Geometry: final body of the model. Coordinates: model frame, mm. Face numbers are marked on the shaded views. A direction names the side the tool comes from. Round coordinates to 2 decimals unless told otherwise and drop trailing zeros. Order: outer loops, then holes, each group sorted by start corner. A loop starts at its lowest first (then second) coordinate and runs counter-clockwise, first axis right, second up. Notation, with made-up numbers: (40, -17.75) - (81, -17.75) arc R9 ccw to (81, -3.75) - close; hole circle Ø5 at (0, 8.25). An arc over 180 degrees is marked (long way). Put each result on its own line as item: value. Start each with the question number.
(1) Section B-B (x = 10). Output: boundary loops of the cut face in (y, z), and give its area (3 significant figures).
(2) Access query for the marked faces 1, 2 and 3. Directions: +Z, -Z, +X, -X, +Y, -Y. A direction counts if a zero-diameter tool reaches every point of the face in a straight line with its end or side. Return the directions, or none.
(3) Section C-C (y = 4.75). Output: boundary loops of the cut face in (x, z).
(4) Section A-A (z = -10.5). Output: boundary loops of the cut face in (x, y).
(5) Material intervals for L1, parallel to X at y = 10, z = -7.75; L2, parallel to Y at x = -6, z = -11.25; L3, parallel to Y at x = -2, z = 11, sorted ascending. Write a range as [from, to].
(6) Pull-direction query (Y, two-part tool) for the marked faces 4, 5 and 6; classes: released by +Y, released by -Y, zero draft, split by the parting line, or undercut.
(7) Pin query (flat end, axial travel): P1, Ø0.5, axis at x = 21.5, y = 13.5, coming from the +Z side; P2, Ø1.5, axis at x = -18.5, z = 4, coming from the +Y side; P3, Ø1.4, axis at x = -22, y = 15.5, coming from the -Z side. Return the tip coordinate at first contact, or that it passes through.
(8) Section D-D (x = 17). Output: boundary loops of the cut face in (y, z).
from build123d import *

# Parameters (mm, degrees)
SKETCH3_W           = 47.5
SKETCH3_H           = 28.7
BOSS_EXTRUDE2_DEPTH = 2.8
SKETCH4_W           = 45
SKETCH4_H           = 25.9
BOSS_EXTRUDE3_DEPTH = 15.6
SKETCH5_W           = 24.9
SKETCH5_H           = 7.77
CUT_EXTRUDE1_DEPTH  = 12.95
SKETCH6_W           = 41.56
SKETCH6_H           = 22.38
CUT_EXTRUDE2_DEPTH  = 4.9
SKETCH7_W           = 1.37
SKETCH7_H           = 11.5
SKETCH7_W_2         = 1.364312096
SKETCH7_W_3         = 5.86
SKETCH7_H_2         = 2.2
CUT_EXTRUDE4_DEPTH  = 1.73


with BuildPart() as part:
    # Sketch3 → Boss-Extrude2 (new body)
    with BuildSketch(Plane(origin=(0, 0, 0), x_dir=(1, 0, 0), z_dir=(0, 1, 0))):
        Rectangle(SKETCH3_W, SKETCH3_H)
    extrude(amount=BOSS_EXTRUDE2_DEPTH)

    # Sketch4 → Boss-Extrude3 (add)
    with BuildSketch(Plane(origin=(0, 2.8, 0), x_dir=(1, 0, 0), z_dir=(0, 1, 0))):
        Rectangle(SKETCH4_W, SKETCH4_H)
    extrude(amount=BOSS_EXTRUDE3_DEPTH)

    # Sketch5 → Cut-Extrude1 (cut)
    with BuildSketch(Plane.XY):
        with Locations((0, 6.685)):
            Rectangle(SKETCH5_W, SKETCH5_H)
    cut_extrude1 = extrude(amount=-CUT_EXTRUDE1_DEPTH, mode=Mode.SUBTRACT)

    # Mirror1: Cut-Extrude1 across plane
    add(cut_extrude1.mirror(Plane.XY), mode=Mode.SUBTRACT)

    # Sketch6 → Cut-Extrude2 (cut)
    with BuildSketch(Plane(origin=(0, 18.4, 0), x_dir=(1, 0, 0), z_dir=(0, 1, 0))):
        Rectangle(SKETCH6_W, SKETCH6_H)
    extrude(amount=-CUT_EXTRUDE2_DEPTH, mode=Mode.SUBTRACT)

    # Sketch7 → Cut-Extrude4 (cut)
    with BuildSketch(Plane(origin=(22.5, 0, 0), x_dir=(0, 0, -1), z_dir=(1, 0, 0))):
        with Locations((5.625, 12.65)):
            Rectangle(SKETCH7_W, SKETCH7_H)
        with Locations((10.417843952, 12.65)):
            Rectangle(SKETCH7_W_2, SKETCH7_H)
        with Locations((0, 12.35)):
            Rectangle(SKETCH7_W_3, SKETCH7_H_2)
        with Locations((-5.625, 12.65)):
            Rectangle(SKETCH7_W, SKETCH7_H)
        with Locations((-10.417843952, 12.65)):
            Rectangle(SKETCH7_W_2, SKETCH7_H)
    cut_extrude4 = extrude(amount=-CUT_EXTRUDE4_DEPTH, mode=Mode.SUBTRACT)

    # Mirror2: Cut-Extrude4 across plane
    add(cut_extrude4.mirror(Plane(origin=(0, 0, 0), x_dir=(0, 0, 1), z_dir=(1, 0, 0))), mode=Mode.SUBTRACT)


solid = part.part
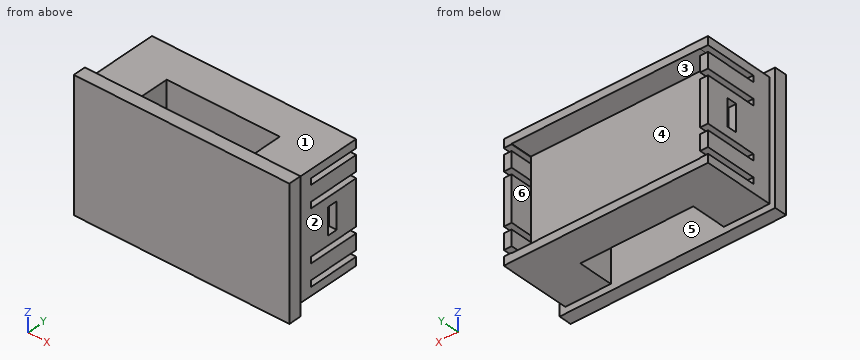
Checks:
1. outline: (0, -14.35) - (2.8, -14.35) - (2.8, 14.35) - (0, 14.35) - close; (10.57, -12.95) - (18.4, -12.95) - (18.4, -11.19) - (13.5, -11.19) - (13.5, 11.19) - (18.4, 11.19) - (18.4, 12.95) - (10.57, 12.95) - close
1. area: 173 mm²
2. face 1: +Z, +X, -X, +Y
2. face 2: +Z, -Z, +X, +Y
2. face 3: +Y
3. outline: (-22.5, -12.95) - (-12.45, -12.95) - (-12.45, 12.95) - (-22.5, 12.95) - close; (12.45, -12.95) - (22.5, -12.95) - (22.5, 12.95) - (12.45, 12.95) - close
4. outline: (-23.75, 0) - (23.75, 0) - (23.75, 2.8) - (22.5, 2.8) - (22.5, 6.9) - (20.77, 6.9) - (20.77, 13.5) - (-20.77, 13.5) - (-20.77, 6.9) - (-22.5, 6.9) - (-22.5, 2.8) - (-23.75, 2.8) - close; hole (-12.45, 2.8) - (12.45, 2.8) - (12.45, 10.57) - (-12.45, 10.57) - close
5. L1: x = [-22.5, -12.45], [12.45, 22.5]
5. L2: y = [0, 2.8], [10.57, 18.4]
5. L3: y = [0, 2.8], [10.57, 13.5]
6. face 4: released by +Y
6. face 5: undercut
6. face 6: zero draft
7. P1: stops at z = 12.95
7. P2: stops at y = 13.5
7. P3: stops at z = -12.95
8. outline: (0, -14.35) - (2.8, -14.35) - (2.8, -12.95) - (18.4, -12.95) - (18.4, -11.19) - (13.5, -11.19) - (13.5, 11.19) - (18.4, 11.19) - (18.4, 12.95) - (2.8, 12.95) - (2.8, 14.35) - (0, 14.35) - close
